```python
from build123d import *

# Parameters (mm, degrees)
F2_W     = 16
F2_H     = 16
F3_DEPTH = 100
F4_W     = 20
F4_H     = 140
F5_DEPTH = 12.5
F6_W     = 16
F6_H     = 20
F7_DEPTH = 25
F9_D     = 4.2


with BuildPart() as f1:
    # F0 (on Front) → F1 (revolve)
    with BuildSketch(Plane.XZ):
        with BuildLine():
            Line((0, -89), (0, 89))
            ThreePointArc((0, 89), (-89, 0), (0, -89))
        make_face()
    revolve(axis=Axis((0, 0, 0), (0, 0, -1)))

    # F2 (on Top) → F3 (intersect, symmetric)
    with BuildSketch(Plane.XY):
        Rectangle(F2_W, F2_H)
    extrude(amount=F3_DEPTH, both=True, mode=Mode.INTERSECT)

    # F4 (on Front) → F5 (cut, symmetric)
    with BuildSketch(Plane.XZ):
        with Locations((0, -30)):
            Rectangle(F4_W, F4_H)
    extrude(amount=F5_DEPTH, both=True, mode=Mode.SUBTRACT)

    # F6 (on Right) → F7 (cut)
    with BuildSketch(Plane.YZ):
        with Locations((0, 50)):
            Rectangle(F6_W, F6_H)
    extrude(amount=-F7_DEPTH, mode=Mode.SUBTRACT)

    # F9 (through all)
    with Locations(Plane(origin=(0, 0, 0), x_dir=(0, -1, 0), z_dir=(-1, 0, 0))):
        with Locations((0, 50)):
            Hole(F9_D / 2)


solid = f1.part
```
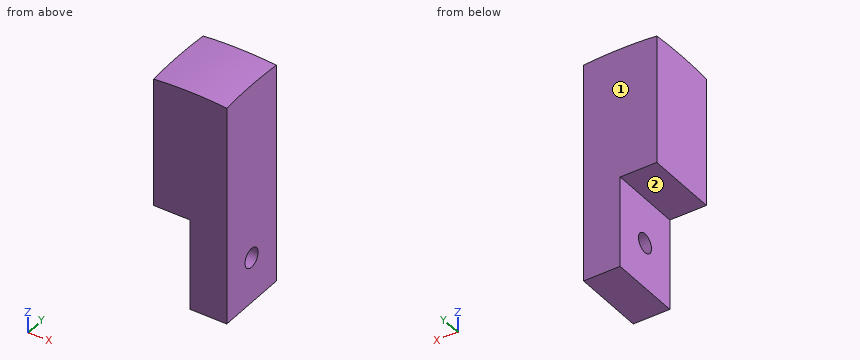
Work out the finished part from the listing and answer in its coordinate system (mm). Face numbers are marked on the shaded views. A direction names the side the tool comes from. Coordinates: 2 decimals unless noted, no trailing zeros. Write each loop counter-clockwise with the first axis right and the second up, starting at its lowest first coordinate (ties: lowest second). Pieces come first, ordered by that corner, then holes.
Q1. A cutting plane is placed at A-A, the plane y = 0. Give the vertices of the cut face in (x, z).
Q2. A cutting plane is placed at B-B, the plane z = 50. Give the vertices of the cut face in (x, y).
Q3. Find the intervals of material crossed by line 1 (X direction, y = 6.5, z = 45.5); line 2 (Z direction, x = 5, y = 0); line 3 (Z direction, x = 6, y = -1.5), in increasing order.
Q4. A cutting plane is placed at C-C, the plane x = 5.75. Give the vertices of the cut face in (y, z).
Q5. A cutting plane is placed at D-D, the plane z = 59. Give the vertices of the cut face in (x, y), then the cut area to 3 significant figures.
Q6. This flat-tipped pin is pushed along its axis until it touches: pin 1 Ø5 at (x, y) = (3.5, 0.5) entering from +Z. Where does it stop, or does it pass through?
Q7. Which of the six approach directions +Z, -Z, +X, -X, +Y, -Y give full straight-line access (tool end or side, diameter ignored) to the marked faces 1 and 2?
Findings below:
1. outline: (-8, 60) - (0, 60) - (0, 52.1) - (8, 52.1) - (8, 88.64) arc R89 ccw to (-8, 88.64) - close; (0, 40) - (8, 40) - (8, 47.9) - (0, 47.9) - close
2. outline: (0, -8) - (8, -8) - (8, -2.1) - (0, -2.1) - close; (0, 2.1) - (8, 2.1) - (8, 8) - (0, 8) - close
3. line 1: x = 0 to 8
3. line 2: z = 40 to 47.9, 52.1 to 88.86
3. line 3: z = 40 to 48.53, 51.47 to 88.78
4. outline: (-8, 40) - (8, 40) - (8, 88.45) arc R88.81 ccw to (-8, 88.45) - close; hole circle Ø4.2 at (0, 50)
5. outline: (0, -8) - (8, -8) - (8, 8) - (0, 8) - close
5. area: 128 mm2
6. pin 1: stops at z = 88.99
7. face 1: +Z, -Z, +X, -X, +Y
7. face 2: -Z, -X, +Y, -Y
